```python
from build123d import *


with BuildPart() as part:
    # Skica1 → Rotovat3 (revolve)
    with BuildSketch(Plane(origin=(0, 0, 0), x_dir=(1, 0, 0), z_dir=(0, 1, 0))):
        Polygon((0, 0), (0, 12.5), (32, 12.5), (32, 15), (51.019237886, 15), (51.019237886, 0), align=None)
    revolve(axis=Axis((-26.278850793, 0, 0), (1, 0, 0)))

    # Skica1_4 → Rotovat4 (revolve)
    with BuildSketch(Plane(origin=(0, 0, 0), x_dir=(1, 0, 0), z_dir=(0, 1, 0))):
        with BuildLine():
            ThreePointArc((101.366985862, 17.5), (107, 0), (101.366985862, -17.5))
            Line((101.366985862, -17.5), (92, -17.5))
            Line((92, -17.5), (92, 17.5))
            Line((92, 17.5), (101.366985862, 17.5))
        make_face()
    revolve(axis=Axis((77, 0, -76.152073434), (0, 0, 1)))


solid = part.part
```
Geometry check sheet. Reference: the model listing, model coordinates, mm. A direction names the side the tool comes from. Coordinates: 2 decimals unless noted, no trailing zeros. Order: outer loops, then holes, each group sorted by start corner. A loop starts at its lowest first (then second) coordinate and runs counter-clockwise, first axis right, second up. Notation, with made-up numbers: M 58,-23 L 113,-23 A22 ccw 113,-6 Z; hole C 13,-35 d5. An arc over 180 degrees is marked long. One line per question, with ' | ' between items. Start each with the question number.
Item 1: Gauge pin test, flat ends, axial feed: pin 1 (1.5 mm diameter, centred on y = -11.5, z = 2.5, fed in from -X); pin 2 (24 mm diameter, centred on x = 77, y = 0, fed in from +Z); pin 3 (1 mm diameter, centred on x = 42, z = -4, fed in from -Y); pin 4 (4 mm diameter, centred on x = 43, z = 13, fed in from -Y). Record the tip position at first contact, or that the pin passes through.
Item 2: Cross-section at C-C on z = 0. Enter the section's corners in (x, y).
Item 3: Cross-section at B-B on x = 77. Enter the section's corners in (y, z), then the cut area to 3 significant figures.
Item 4: Cross-section at D-D on x = 19. Enter the section's corners in (y, z), then the cut area to 3 significant figures.
Item 5: Set-up check for faces 4 (the cylindrical face through (41.643, 0.66, 14.985)), 5 (the flat face through (66.5, 11.2, -17.5)): record each of +Z, -Z, +X, -X, +Y, -Y from which the full face is reachable in a straight line by a thin tool's end or side.
Item 6: Cross-section at A-A on y = 0. Enter the section's corners in (x, z).
Item 7: Draft check along X on faces 1 (the flat face through (0, 0, 0)), 2 (the cylindrical face through (16.224, 3.755, -11.923)), 3 (the cylindrical face through (62.015, 0.66, -0.245)). Enter one of: pulls with the +X half, pulls with the -X half, needs draft (parallel to the pull), parting line crosses it, or undercut.
Item 8: Material ranges on L1, parallel to Y at x = 77, z = 9; L2, parallel to Y at x = 64.5, z = -5.5; L3, parallel to X at y = 11.5, z = -10, recorded low to high. Write a range as [from, to].
Findings:
1) pin 1: stops at x = 0 | pin 2: passes through | pin 3: stops at y = -14.59 | pin 4: stops at y = -10.2
2) outline: M 0,-12.5 L 32,-12.5 L 32,-15 L 51.02,-15 A30 ccw long 51.02,15 L 32,15 L 32,12.5 L 0,12.5 Z; hole C 77,0 d30
3) outline: M -24.37,-17.5 L -15,-17.5 L -15,17.5 L -24.37,17.5 A30 ccw Z; M 15,-17.5 L 24.37,-17.5 A30 ccw 24.37,17.5 L 15,17.5 Z | area: 924 mm²
4) outline: C 0,0 d25 | area: 491 mm²
5) face 4: -X | face 5: -Z, +X, -X, +Y, -Y
6) outline: M 0,-12.5 L 32,-12.5 L 32,-15 L 51.02,-15 A30 ccw 52.63,-17.5 L 62,-17.5 L 62,17.5 L 52.63,17.5 A30 ccw 51.02,15 L 32,15 L 32,12.5 L 0,12.5 Z; M 92,-17.5 L 101.37,-17.5 A30 ccw 101.37,17.5 L 92,17.5 Z
7) face 1: pulls with the -X half | face 2: needs draft | face 3: undercut
8) L1: y = [-28.62, -15], [15, 28.62] | L2: y = [-26.71, -8.29], [8.29, 26.71] | L3: x = [51.16, 67.37], [86.63, 102.84]
